Geometry: final body of the model. Coordinates: model frame, mm. Give positions to 0.01 mm unless a question says otherwise; leave off trailing zeros. Order: outer loops, then holes, each group sorted by start corner. A loop starts at its lowest first (then second) coordinate and runs counter-clockwise, first axis right, second up. Notation, with made-up numbers: (46, 79.25) - (90, 79.25) arc R19 ccw to (90, 90.25) - close; hole circle Ø8 at (43, 52). An arc over 180 degrees is marked (long way). One line per item, written item: value.
```python
from build123d import *

# Parameters (mm, degrees)
F0_R          = 12.7
F1_DEPTH      = 3.175
F2_R          = 1.5875
F3_DEPTH      = 14.351
F3_DEPTH_BACK = 14.351
F4_R          = 1.27
F5_SIZE       = 0.762


with BuildPart() as f1:
    # F0 (on Top) → F1 (new body, symmetric)
    with BuildSketch(Plane.XY):
        Circle(F0_R)
    extrude(amount=F1_DEPTH, both=True)

    # F2 (on Right) → F3 (join, two sides)
    with BuildSketch(Plane.YZ) as f3_sk:
        Circle(F2_R)
    extrude(amount=-F3_DEPTH)
    extrude(f3_sk.sketch, amount=F3_DEPTH_BACK)

    # F4
    f4_edges = [f1.edges().sort_by_distance(p)[0] for p in [
        (-14.351, -1.5875, 0),
        (14.351, -1.5875, 0),
    ]]
    fillet(f4_edges, radius=F4_R)

    # F5
    f5_edges = [f1.edges().sort_by_distance(p)[0] for p in [
        (-12.7, 0, 3.175),
        (-12.7, 0, -3.175),
    ]]
    chamfer(f5_edges, length=F5_SIZE)


solid = f1.part
```
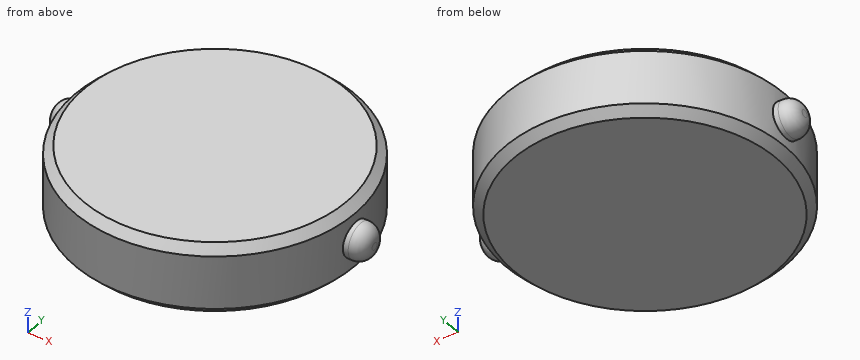
1) First-contact query: pin 1 (1.5 mm diameter, centred on x = -10.5, y = 7.5, fed in from -Z); pin 2 (2 mm diameter, centred on x = 1.5, z = -0.5, fed in from +Y). Flat tips, straight axial feed; report the tip coordinate or a pass-through.
Answers below:
pin 1: z = -2.96
pin 2: y = 12.69
2) Section A-A, the plane z = 2. Return loops of the section in (x, y).
Answers below:
outline: circle Ø25.4 at (0, 0)
3) Material intervals for line 1 along X through (y, z) = (-8.75, -0.5); line 2 along X through (y, z) = (11, 1.5); line 3 along Y through (x, z) = (7, 2.75), sorted ascending.
Answers below:
line 1: -9.2 to 9.2
line 2: -6.35 to 6.35
line 3: -10.19 to 10.19
